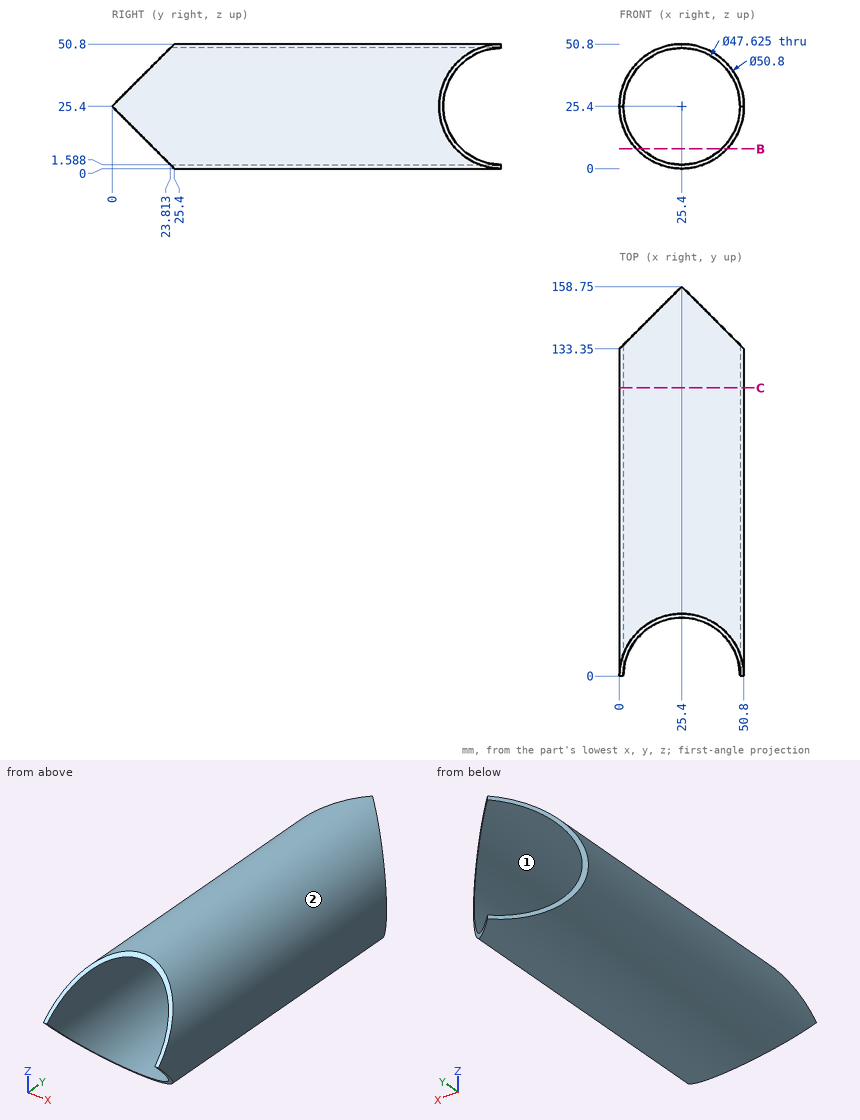
Print and shaded views of the part. All mm, measured from the part's lowest x, y and z. Round coordinates to 2 decimals unless told otherwise and drop trailing zeros. Order: outer loops, then holes, each group sorted by start corner. A loop starts at its lowest first (then second) coordinate and runs counter-clockwise, first axis right, second up.
Q1. Wall check: L1, parallel to X at y = 64, z = 25.4; L2, parallel to Z at x = 8.5, y = 17 (1 decimal). Give the ranges that are in metal, low to high.
Q2. Slice it at C-C (y = 117.5). Write the cut outline in (x, z) (1 decimal).
Q3. Slice it at B-B (z = 8). Write the cut outline in (x, y) (1 decimal).
Q4. Two-plate mould, pull along Z, no slides. Class the marked faces 1 and 2: pulls with the +Z half, pulls with the -Z half, needs draft (parallel to the pull), parting line crosses it, or undercut.
Q5. Drop flat-ended pins along their axis: pin 1 (8 mm diameter, centred on y = 79.5, z = 21, fed in from +X); pin 2 (1.5 mm diameter, centred on y = 72, z = 6.5, fed in from -X); pin 3 (8 mm diameter, centred on x = 5, y = 85.5, fed in from -Z) (1 decimal). Give the stop position or say it passes through.
Results below:
1. L1: x = 0 to 1.59, 49.21 to 50.8
1. L2: z = 8.4 to 8.6, 42.2 to 42.4
2. outline: circle Ø50.8 at (25.4, 25.4); hole circle Ø47.6 at (25.4, 25.4)
3. outline: (6.9, 17.4) - (9.1, 17.4) - (9.1, 142.5) - (6.9, 140.2) - close; (41.7, 17.4) - (43.9, 17.4) - (43.9, 140.2) - (41.7, 142.5) - close
4. face 1: undercut
4. face 2: parting line crosses it
5. pin 1: stops at x = 50.8
5. pin 2: stops at x = 7.63
5. pin 3: stops at z = 6
